Can you work these out from the model? Positions are in its coordinate system, mm. Face numbers are marked on the shaded views. A direction names the side the tool comes from. Give positions to 0.01 mm unless a question says otherwise; leave off trailing zeros. Loops run counter-clockwise (first coordinate to the right, second up) from the corner with the lowest first, then second, coordinate; pieces in that order, holes last. Notation, with made-up numbers: (-3.5, 55) - (27.5, 55) arc R10 ccw to (27.5, 61) - close; hole circle Ø8 at (-9.5, 30.25). An arc over 180 degrees is marked (long way). Answer as a JSON object with one key per item and string values.
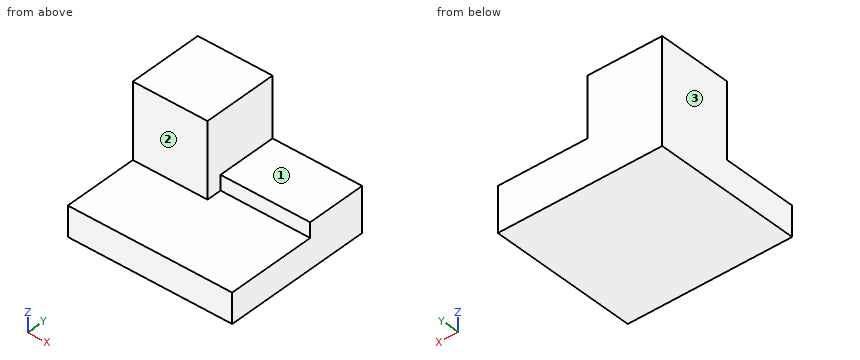
```python
from build123d import *

# Parameters (mm, degrees)
F0_W     = 55
F0_H     = 10
F1_DEPTH = 50
F3_W     = 20
F3_H     = 15
F4_DEPTH = 55
F2_W     = 25
F2_H     = 25
F5_DEPTH = 25


with BuildPart() as f1:
    # F0 (on Front) → F1 (new body)
    with BuildSketch(Plane.XZ):
        Rectangle(F0_W, F0_H)
    extrude(amount=F1_DEPTH)

    # F3 (on face) → F4 (join)
    with BuildSketch(Plane.YZ.offset(27.5)):
        with Locations((-10, 2.5)):
            Rectangle(F3_W, F3_H)
    extrude(amount=-F4_DEPTH)

    # F2 (on face) → F5 (join)
    with BuildSketch(Plane.XY.offset(5)):
        with Locations((-15, -12.5)):
            Rectangle(F2_W, F2_H)
    extrude(amount=F5_DEPTH)


solid = f1.part
```
1) Imagine slicing it at D-D on y = -42. Write out the boundary of the cut face in (x, z), and give its area (3 significant figures).
Check sheet entries:
{"outline": "(-27.5, -5) - (27.5, -5) - (27.5, 5) - (-27.5, 5) - close", "area": "550 mm2"}
2) Imagine slicing it at C-C on z = 23.5. Write out the boundary of the cut face in (x, y), and give its area (3 significant figures).
Check sheet entries:
{"outline": "(-27.5, -25) - (-2.5, -25) - (-2.5, 0) - (-27.5, 0) - close", "area": "625 mm2"}
3) Imagine slicing it at A-A on x = 14.5. Write out the boundary of the cut face in (y, z).
Check sheet entries:
{"outline": "(-50, -5) - (0, -5) - (0, 10) - (-20, 10) - (-20, 5) - (-50, 5) - close"}
4) I'm going to push flat-ended pins straight in: P1, Ø20, axis at y = -14.5, z = 15.5, coming from the +X side; P2, Ø1.5, axis at x = -7.5, y = -40.5, coming from the +Z side; P3, Ø8, axis at y = -16.5, z = 19, coming from the +X side; P4, Ø6, axis at x = 1, z = 23, coming from the +Y side. Where does each tip first touch, or does it pass through?
Check sheet entries:
{"P1": "x = 27.5", "P2": "z = 5", "P3": "x = -2.5", "P4": "through"}
5) Which directions (+Z, -Z, +X, -X, +Y, -Y) give clear straight access to the entire face, cutting with the end or side of a thin tool? Please do the marked faces 1, 2 and 3.
Check sheet entries:
{"face 1": "+Z, +X, +Y, -Y", "face 2": "+Z, +X, -X, -Y", "face 3": "+Z, -Z, -X, +Y, -Y"}
6) I need wall thicknesses on L1, parallel to Z at x = 3.5, y = -6.5; L2, parallel to X at y = -24, z = 17; L3, parallel to Z at x = -4, y = -32. Which ranges of each line are inside material? Lowest first, please.
Check sheet entries:
{"L1": "-5 to 10", "L2": "-27.5 to -2.5", "L3": "-5 to 5"}
7) Imagine slicing it at B-B on y = -17.5. Write out the boundary of the cut face in (x, z), and give its area (4 significant figures).
Check sheet entries:
{"outline": "(-27.5, -5) - (27.5, -5) - (27.5, 10) - (-2.5, 10) - (-2.5, 30) - (-27.5, 30) - close", "area": "1,325 mm2"}
